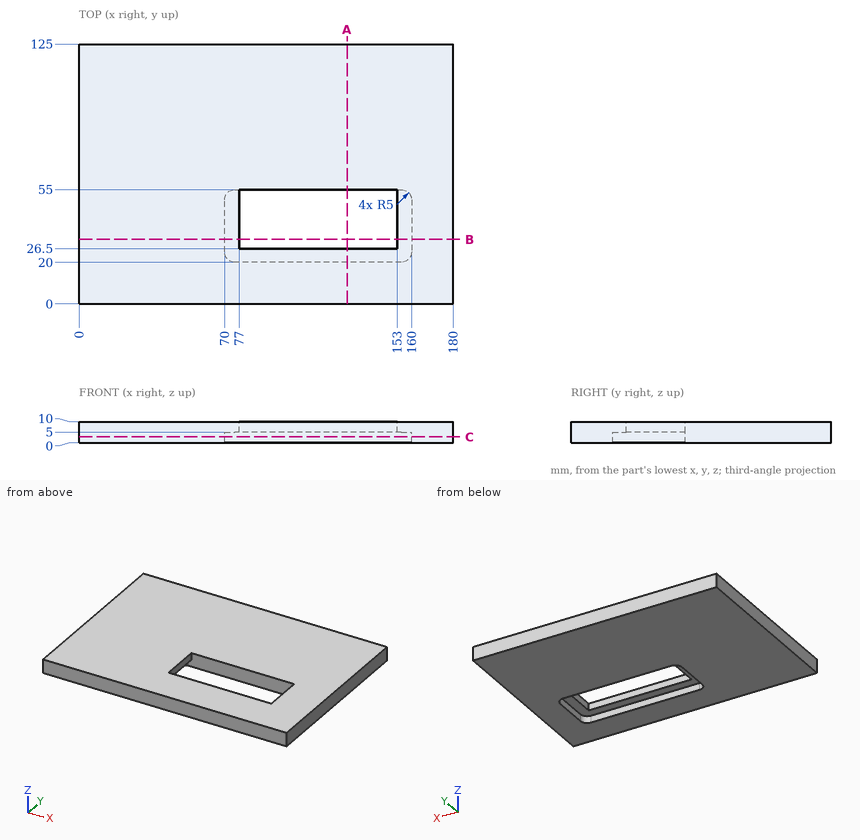
Source: three-view drawing plus pictorial views. Frame: mm from the lowest corner of the part. Give positions to 0.01 mm unless a question says otherwise; leave off trailing zeros. Order: outer loops, then holes, each group sorted by start corner. A loop starts at its lowest first (then second) coordinate and runs counter-clockwise, first axis right, second up. Notation, with made-up numbers: (41, 87.25) -> (58, 87.25) arc R18 cw to (58, 118.25) -> close; hole circle Ø2 at (33, 61). An arc over 180 degrees is marked (long way). Put each result on its own line as item: value.
Q1. Section B-B, the plane y = 31. Return loops of the section in (x, z), then the cut area to 3 significant figures.
Here are the results:
outline: (0, 0) -> (70, 0) -> (70, 5) -> (77, 5) -> (77, 10) -> (0, 10) -> close; (153, 5) -> (160, 5) -> (160, 0) -> (180, 0) -> (180, 10) -> (153, 10) -> close
area: 970 mm^2
Q2. Section C-C, the plane z = 2.75. Return loops of the section in (x, y).
Here are the results:
outline: (0, 0) -> (180, 0) -> (180, 125) -> (0, 125) -> close; hole (70, 25) arc R5 ccw to (75, 20) -> (155, 20) arc R5 ccw to (160, 25) -> (160, 50) arc R5 ccw to (155, 55) -> (75, 55) arc R5 ccw to (70, 50) -> close
Q3. Section A-A, the plane x = 129. Return loops of the section in (y, z).
Here are the results:
outline: (0, 0) -> (20, 0) -> (20, 5) -> (26.5, 5) -> (26.5, 10) -> (0, 10) -> close; (55, 0) -> (125, 0) -> (125, 10) -> (55, 10) -> close
Q4. Material intervals for L1, parallel to Y at x = 84, z = 3.75; L2, parallel to X at y = 37, z = 3.5; L3, parallel to Y at x = 158.5, z = 4.5, sorted ascending.
Here are the results:
L1: y = 0 to 20, 55 to 125
L2: x = 0 to 70, 160 to 180
L3: y = 0 to 21.43, 53.57 to 125
